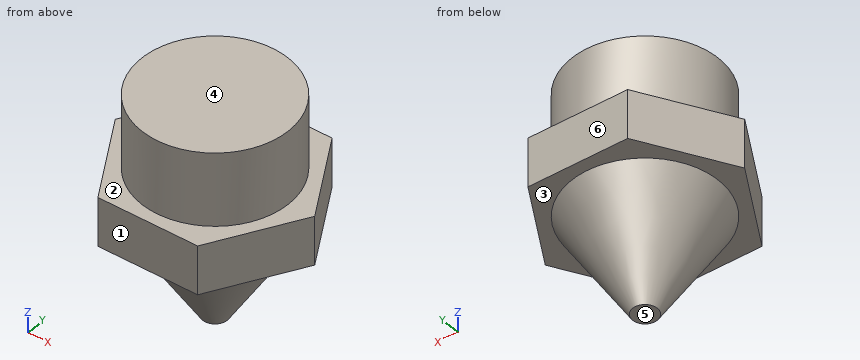
```python
from build123d import *

# Parameters (mm, degrees)
BOSS_EXTRU_1_DEPTH      = 9
ESQUISSE2_W             = 19.623971562
ESQUISSE2_H             = 15.534154535
ESQUISSE2_R             = 3
ENL_V_MAT_EXTRU_1_DEPTH = 3
ENL_V_START             = -4
ESQUISSE3_W             = 11.267201257
ESQUISSE3_H             = 13.961169169
ESQUISSE3_R             = 3
ENL_V_MAT_EXTRU_2_DEPTH = 4
CHANFREIN1_SIZE         = 4
CHANFREIN1_SIZE_2       = 2.499477408


with BuildPart() as part:
    # Esquisse1 → Boss.-Extru.1 (new body)
    with BuildSketch(Plane.XY):
        Polygon((4.041451884, 0), (2.020725942, 3.5), (-2.020725942, 3.5), (-4.041451884, 0), (-2.020725942, -3.5), (2.020725942, -3.5), align=None)
    extrude(amount=BOSS_EXTRU_1_DEPTH)

    # Esquisse2 → Enlèv. mat.-Extru.1 (cut)
    with BuildSketch(Plane.XY.offset(9)):
        with Locations((0.327116653, -1.544441398)):
            Rectangle(ESQUISSE2_W, ESQUISSE2_H)
        Circle(ESQUISSE2_R, mode=Mode.SUBTRACT)
    extrude(amount=-ENL_V_MAT_EXTRU_1_DEPTH, mode=Mode.SUBTRACT)

    # Esquisse3 → Enlèv. mat.-Extru.2 (cut)
    with BuildSketch(Plane(origin=(0, 0, 0), x_dir=(-1, 0, 0), z_dir=(0, 0, -1)).offset(ENL_V_START)):
        with Locations((0.009770186, 0.039262349)):
            Rectangle(ESQUISSE3_W, ESQUISSE3_H)
        with Locations(Location((0, 0, 0), (0, 0, 180))):
            Circle(ESQUISSE3_R, mode=Mode.SUBTRACT)
    extrude(amount=ENL_V_MAT_EXTRU_2_DEPTH, mode=Mode.SUBTRACT)

    # Chanfrein1
    # the kernel refuses this chamfer: 4, 2.499477408 mm, written as the material it takes off along each edge
    with BuildSketch(Plane(origin=(0, 0, 0), x_dir=(1, 0, 0), z_dir=(0, 1, 0))) as chanfrein1_piece_1_section:
        Polygon((3, -CHANFREIN1_SIZE), (3 - CHANFREIN1_SIZE_2, 0), (3, 0), align=None)
    chanfrein1_piece_1 = revolve(axis=Axis((0, 0, 0), (0, 0, -1)), mode=Mode.PRIVATE)
    chanfrein1_piece_1 = split(chanfrein1_piece_1, bisect_by=Plane(origin=(-1.744026904, 0, 4), z_dir=(0, 0, -1)), keep=Keep.TOP, mode=Mode.PRIVATE)
    add(chanfrein1_piece_1, mode=Mode.SUBTRACT)


solid = part.part
```
The listing builds one solid part. Answer for the finished solid, in the listing's coordinates (mm). Face numbers are marked on the shaded views. A direction names the side the tool comes from. Round coordinates to 2 decimals unless told otherwise and drop trailing zeros. Write each loop counter-clockwise with the first axis right and the second up, starting at its lowest first coordinate (ties: lowest second). Pieces come first, ordered by that corner, then holes. Notation, with made-up numbers: (-4.75, -24) -> (30.25, -24) arc R28 ccw to (30.25, 8) -> close; hole circle Ø9 at (59, 10.25). An arc over 180 degrees is marked (long way). Write item = value, one per line.
1) Given pin 1 (1.5 mm diameter, centred on y = -1.5, z = 6, fed in from +X); pin 2 (4 mm diameter, centred on x = -3, y = 0, fed in from -Z); pin 3 (1 mm diameter, centred on y = 1, z = 4.5, fed in from +X), each flat-ended and moving along its own axis, determine where each tip first touches the part or whether it passes through.
Check values:
pin_1 = 3.61
pin_2 = 0.8
pin_3 = 3.75
2) Section B-B on z = 5 is taken. Write down the section's boundary in (x, y).
Check values:
outline = (-4.04, 0) -> (-2.02, -3.5) -> (2.02, -3.5) -> (4.04, 0) -> (2.02, 3.5) -> (-2.02, 3.5) -> close
3) Section D-D on x = -3.5 is taken. Write down the section's boundary in (y, z).
Check values:
outline = (-0.94, 4) -> (0.94, 4) -> (0.94, 6) -> (-0.94, 6) -> close
4) For a pull along Z with two mould halves and no side action, classify the marked faces 4, 5 and 6 as released by +Z, released by -Z, zero draft, split by the parting line, or undercut.
Check values:
face_4 = released by +Z
face_5 = released by -Z
face_6 = zero draft
5) Section A-A on x = 0 is taken. Write down the section's boundary in (y, z).
Check values:
outline = (-3.5, 4) -> (-3, 4) -> (-0.5, 0) -> (0.5, 0) -> (3, 4) -> (3.5, 4) -> (3.5, 6) -> (3, 6) -> (3, 9) -> (-3, 9) -> (-3, 6) -> (-3.5, 6) -> close
6) Straight lines are drawn through the part: line 1 along Z through (x, y) = (2.25, -3); line 2 along Y through (x, z) = (2.75, 6.5); line 3 along Z through (x, y) = (-1.75, -2). For each, find the intervals that lie inside material, in ascending order. Write a range as [from, to].
Check values:
line_1 = [4, 6]
line_2 = [-1.2, 1.2]
line_3 = [3.45, 9]
7) Section C-C on z = 7.75 is taken. Write down the section's boundary in (x, y).
Check values:
outline = circle Ø6 at (0, 0)
8) Which of the six approach directions +Z, -Z, +X, -X, +Y, -Y give full straight-line access (tool end or side, diameter ignored) to the marked faces 1, 2 and 3?
Check values:
face_1 = +Z, -Z, +X, -X, -Y
face_2 = +Z
face_3 = -Z
